```python
from build123d import *

# Parameters (mm, degrees)
F0_W     = 700
F0_H     = 650
F1_DEPTH = 440
F3_DEPTH = 440.001
F4_W     = 140
F4_H     = 250
F5_DEPTH = 120


with BuildPart() as f1:
    # F0 (on Front) → F1 (new body)
    with BuildSketch(Plane.XZ):
        Rectangle(F0_W, F0_H)
    extrude(amount=F1_DEPTH)

    # F2 (on face) → F3 (cut, through all)
    with BuildSketch(Plane.XZ.offset(440)):
        Polygon((-150, -325), (-350, 75), (-350, -325), align=None)
        Polygon((350, 75), (150, -325), (350, -325), align=None)
    extrude(amount=-F3_DEPTH, mode=Mode.SUBTRACT)

    # F4 (on face) → F5 (join)
    with BuildSketch(Plane.XY.offset(325)):
        with Locations((420, -125)):
            Rectangle(F4_W, F4_H)
        with Locations((-420, -125)):
            Rectangle(F4_W, F4_H)
    extrude(amount=-F5_DEPTH)


solid = f1.part
```
The listing builds one solid part. Answer for the finished solid, in the listing's coordinates (mm). A direction names the side the tool comes from. Round coordinates to 2 decimals unless told otherwise and drop trailing zeros. Loops run counter-clockwise (first coordinate to the right, second up) from the corner with the lowest first, then second, coordinate; pieces in that order, holes last. Notation, with made-up numbers: (44, 45) -> (62, 45) arc R12 cw to (62, 66) -> close; hole circle Ø1 at (-1.75, -16). An arc over 180 degrees is marked (long way). Use one line per item in the form item = value.
1. The part is cut by section A-A on z = 243.5. Determine the outline of the cut face in (x, y).
Answer key:
outline = (-490, -250) -> (-350, -250) -> (-350, -440) -> (350, -440) -> (350, -250) -> (490, -250) -> (490, 0) -> (-490, 0) -> close
2. The part is cut by section C-C on x = 200.5. Determine the outline of the cut face in (y, z).
Answer key:
outline = (-440, -224) -> (0, -224) -> (0, 325) -> (-440, 325) -> close
3. The part is cut by section D-D on y = -306. Determine the outline of the cut face in (x, z), and give its area (3 significant figures).
Answer key:
outline = (-350, 75) -> (-150, -325) -> (150, -325) -> (350, 75) -> (350, 325) -> (-350, 325) -> close
area = 375,000 mm²
4. A tool of negligible diameter and unlimited length cuts with its end or side. For faces 1 (the flat face through (419, -250, 266)), 2 (the flat face through (-421, -123, 205)), 3 (the flat face through (-421, -250, 266)), 4 (the flat face through (419, -123, 205)), from which of +Z, -Z, +X, -X, +Y, -Y can it reach the whole face along a straight path? Write none if from no direction.
Answer key:
face_1 = +Z, -Z, +X, -Y
face_2 = -Z, -X, +Y, -Y
face_3 = +Z, -Z, -X, -Y
face_4 = -Z, +X, +Y, -Y
5. The part is cut by section B-B on y = -105. Determine the outline of the cut face in (x, z), and give its area (3 significant figures).
Answer key:
outline = (-490, 205) -> (-350, 205) -> (-350, 75) -> (-150, -325) -> (150, -325) -> (350, 75) -> (350, 205) -> (490, 205) -> (490, 325) -> (-490, 325) -> close
area = 409,000 mm²
6. Find the intervals of material crossed by probe 1 along X at (y, z) = (-280, 81.5); probe 2 along Z at (x, y) = (-214.5, -32); probe 3 along Z at (x, y) = (401, -69), in increasing order. Write a range as [from, to].
Answer key:
probe_1 = [-350, 350]
probe_2 = [-196, 325]
probe_3 = [205, 325]
7. Flat-ended cylindrical pins translate along their axes: pin 1 Ø3 at (x, y) = (-306, -63.5) entering from -Z; pin 2 Ø10 at (y, z) = (-297.5, 109) entering from +X; pin 3 Ø12 at (x, y) = (-160.5, -322.5) entering from -Z; pin 4 Ø12 at (x, z) = (-135.5, 224) entering from +Y. Find the tip coordinate at first contact, or state that the pin passes through.
Answer key:
pin_1 = -16
pin_2 = 350
pin_3 = -316
pin_4 = 0
